Build history of the part. All positions in model axes, mm. Face numbers are marked on the shaded views. A direction names the side the tool comes from. Give positions to 0.01 mm unless a question says otherwise; leave off trailing zeros. Use a Markdown table: item, result. Add a question column.
(1) Flat gauge pins, fed straight in: pin 1 (2 mm diameter, centred on x = 70.5, y = -4.5, fed in from -Z) (3 decimals); pin 2 (1 mm diameter, centred on x = 233.5, z = -1, fed in from +Y). Where does each tip first touch, or does it go through?
(2) Which spindle directions (+Z, -Z, +X, -X, +Y, -Y) get a long thin tool onto all of the face, cutting with end or side? Do the marked faces 1 and 2. Say none if no direction does.
(3) Wall check: line 1 (Y direction, x = 650, z = -1.55); line 2 (Y direction, x = 520, z = -0.65); line 3 (Z direction, x = 351, y = 52.5) (3 decimals). Give the ranges that are in metal, low to high.
from build123d import *

# Parameters (mm, degrees)
SKETCH1_R                    = 11.9875
SKETCH1_R_2                  = 11.1125
SKETCH1_W                    = 75
SKETCH1_H                    = 10.02
BASE_FLANGE1_DEPTH           = 3.175
EDGE_FLANGE1_STRIP_W         = 14.1732
EDGE_FLANGE1_STRIP_H         = 3.175
EDGE_FLANGE1_STRIP_CUT_DEPTH = 910
EDGE_FLANGE1_DEPTH           = 910
M5_CLEARANCE_HOLE1_D         = 5.3
CUT_EXTRUDE2_REACH           = 784.448
FILLET1_R                    = 2
FILLET2_R                    = 5


# Sheet-metal steps are written as plain solids
with BuildPart() as part:
    # Sketch1 → Base-Flange1 (new body)
    with BuildSketch(Plane.XY):
        Polygon((-130, 60), (780, 60), (780, -20), (700, -55), (0, -55), (-130, -20), align=None)
        Circle(SKETCH1_R, mode=Mode.SUBTRACT)
        with Locations((183.333333333, 0)):
            Circle(SKETCH1_R, mode=Mode.SUBTRACT)
        with Locations((366.666666667, 0)):
            Circle(SKETCH1_R, mode=Mode.SUBTRACT)
        with Locations((550, 0)):
            Circle(SKETCH1_R, mode=Mode.SUBTRACT)
        with Locations((-110, 0)):
            Circle(SKETCH1_R_2, mode=Mode.SUBTRACT)
        with Locations((727.5, 0)):
            Rectangle(SKETCH1_W, SKETCH1_H, mode=Mode.SUBTRACT)
    extrude(amount=-BASE_FLANGE1_DEPTH)

    # Edge-Flange1 strip (across the edge) → Edge-Flange1 strip cut (cut)
    with BuildSketch(Plane(origin=(-130, 60, -3.175), x_dir=(0, -1, 0), z_dir=(1, 0, 0))):
        with Locations((-3.175, -1.5875)):
            Rectangle(EDGE_FLANGE1_STRIP_W, EDGE_FLANGE1_STRIP_H)
    extrude(amount=EDGE_FLANGE1_STRIP_CUT_DEPTH, mode=Mode.SUBTRACT)

    # Edge-Flange1 section (across the edge) → Edge-Flange1 (add)
    with BuildSketch(Plane(origin=(-130, 60, -3.175), x_dir=(0, -1, 0), z_dir=(1, 0, 0))):
        with BuildLine():
            Line((0, 0.7366), (0, 11.825))
            Line((0, 11.825), (3.175, 11.825))
            Line((3.175, 11.825), (3.175, 0.7366))
            ThreePointArc((3.175, 0.7366), (3.390745145, 0.215745145), (3.9116, 0))
            Line((3.9116, 0), (3.9116, -3.175))
            ThreePointArc((3.9116, -3.175), (1.145681115, -2.029318885), (0, 0.7366))
        make_face()
    extrude(amount=EDGE_FLANGE1_DEPTH)

    # M5 Clearance Hole1 (through all)
    with Locations(Plane(origin=(-50, 10, 0), x_dir=(1, 0, 0), z_dir=(0, 0, 1))):
        with Locations((0, 0), (0, -20), (20, -35), (20, 15), (183.333333333, 0), (183.333333333, -20), (203.333333333, -35), (203.333333333, 15), (366.666666667, 0), (366.666666667, -20), (386.666666667, -35), (386.666666667, 15), (550, 0), (550, -20), (570, -35), (570, 15), (700, 0), (700, -20), (720, 15), (720, -35)):
            Hole(M5_CLEARANCE_HOLE1_D / 2)

    # Sketch8 → Cut-Extrude2 (cut, up to next)
    with BuildSketch(Plane.XY, mode=Mode.PRIVATE) as cut_extrude2_sk1:
        Polygon((55.816057945, 40), (25, 40), (25, -22.943437506), align=None)
    cut_extrude2_tool1 = extrude(cut_extrude2_sk1.sketch, amount=-CUT_EXTRUDE2_REACH, mode=Mode.PRIVATE) & part.part
    # Sketch8 → Cut-Extrude2 (cut, up to next)
    with BuildSketch(Plane.XY, mode=Mode.PRIVATE) as cut_extrude2_sk2:
        Polygon((64.166666667, -40), (33.350608721, -40), (64.166666667, 22.943437506), align=None)
    cut_extrude2_tool2 = extrude(cut_extrude2_sk2.sketch, amount=-CUT_EXTRUDE2_REACH, mode=Mode.PRIVATE) & part.part
    # Sketch8 → Cut-Extrude2 (cut, up to next)
    with BuildSketch(Plane.XY, mode=Mode.PRIVATE) as cut_extrude2_sk3:
        Polygon((79.166666667, -40), (79.166666667, 22.943437506), (109.982724612, -40), align=None)
    cut_extrude2_tool3 = extrude(cut_extrude2_sk3.sketch, amount=-CUT_EXTRUDE2_REACH, mode=Mode.PRIVATE) & part.part
    # Sketch8 → Cut-Extrude2 (cut, up to next)
    with BuildSketch(Plane.XY, mode=Mode.PRIVATE) as cut_extrude2_sk4:
        Polygon((118.333333333, 40), (118.333333333, -22.943437506), (87.517275388, 40), align=None)
    cut_extrude2_tool4 = extrude(cut_extrude2_sk4.sketch, amount=-CUT_EXTRUDE2_REACH, mode=Mode.PRIVATE) & part.part
    # Sketch8 → Cut-Extrude2 (cut, up to next)
    with BuildSketch(Plane.XY, mode=Mode.PRIVATE) as cut_extrude2_sk5:
        Polygon((239.149391279, 40), (208.333333333, -22.943437506), (208.333333333, 40), align=None)
    cut_extrude2_tool5 = extrude(cut_extrude2_sk5.sketch, amount=-CUT_EXTRUDE2_REACH, mode=Mode.PRIVATE) & part.part
    # Sketch8 → Cut-Extrude2 (cut, up to next)
    with BuildSketch(Plane.XY, mode=Mode.PRIVATE) as cut_extrude2_sk6:
        Polygon((247.5, 22.943437506), (247.5, -40), (216.683942055, -40), align=None)
    cut_extrude2_tool6 = extrude(cut_extrude2_sk6.sketch, amount=-CUT_EXTRUDE2_REACH, mode=Mode.PRIVATE) & part.part
    # Sketch8 → Cut-Extrude2 (cut, up to next)
    with BuildSketch(Plane.XY, mode=Mode.PRIVATE) as cut_extrude2_sk7:
        Polygon((293.316057945, -40), (262.5, -40), (262.5, 22.943437506), align=None)
    cut_extrude2_tool7 = extrude(cut_extrude2_sk7.sketch, amount=-CUT_EXTRUDE2_REACH, mode=Mode.PRIVATE) & part.part
    # Sketch8 → Cut-Extrude2 (cut, up to next)
    with BuildSketch(Plane.XY, mode=Mode.PRIVATE) as cut_extrude2_sk8:
        Polygon((270.850608721, 40), (301.666666667, 40), (301.666666667, -22.943437506), align=None)
    cut_extrude2_tool8 = extrude(cut_extrude2_sk8.sketch, amount=-CUT_EXTRUDE2_REACH, mode=Mode.PRIVATE) & part.part
    # Sketch8 → Cut-Extrude2 (cut, up to next)
    with BuildSketch(Plane.XY, mode=Mode.PRIVATE) as cut_extrude2_sk9:
        Polygon((422.482724612, 40), (391.666666667, -22.943437506), (391.666666667, 40), align=None)
    cut_extrude2_tool9 = extrude(cut_extrude2_sk9.sketch, amount=-CUT_EXTRUDE2_REACH, mode=Mode.PRIVATE) & part.part
    # Sketch8 → Cut-Extrude2 (cut, up to next)
    with BuildSketch(Plane.XY, mode=Mode.PRIVATE) as cut_extrude2_sk10:
        Polygon((430.833333333, 22.943437506), (430.833333333, -40), (400.017275388, -40), align=None)
    cut_extrude2_tool10 = extrude(cut_extrude2_sk10.sketch, amount=-CUT_EXTRUDE2_REACH, mode=Mode.PRIVATE) & part.part
    # Sketch8 → Cut-Extrude2 (cut, up to next)
    with BuildSketch(Plane.XY, mode=Mode.PRIVATE) as cut_extrude2_sk11:
        Polygon((476.649391279, -40), (445.833333333, -40), (445.833333333, 22.943437506), align=None)
    cut_extrude2_tool11 = extrude(cut_extrude2_sk11.sketch, amount=-CUT_EXTRUDE2_REACH, mode=Mode.PRIVATE) & part.part
    # Sketch8 → Cut-Extrude2 (cut, up to next)
    with BuildSketch(Plane.XY, mode=Mode.PRIVATE) as cut_extrude2_sk12:
        Polygon((454.183942055, 40), (485, 40), (485, -22.943437506), align=None)
    cut_extrude2_tool12 = extrude(cut_extrude2_sk12.sketch, amount=-CUT_EXTRUDE2_REACH, mode=Mode.PRIVATE) & part.part
    # Sketch8 → Cut-Extrude2 (cut, up to next)
    with BuildSketch(Plane.XY, mode=Mode.PRIVATE) as cut_extrude2_sk13:
        Polygon((605.816057945, 40), (575, -22.943437506), (575, 40), align=None)
    cut_extrude2_tool13 = extrude(cut_extrude2_sk13.sketch, amount=-CUT_EXTRUDE2_REACH, mode=Mode.PRIVATE) & part.part
    # Sketch8 → Cut-Extrude2 (cut, up to next)
    with BuildSketch(Plane.XY, mode=Mode.PRIVATE) as cut_extrude2_sk14:
        Polygon((614.166666667, 22.943437506), (614.166666667, -40), (583.350608721, -40), align=None)
    cut_extrude2_tool14 = extrude(cut_extrude2_sk14.sketch, amount=-CUT_EXTRUDE2_REACH, mode=Mode.PRIVATE) & part.part
    # Sketch8 → Cut-Extrude2 (cut, up to next)
    with BuildSketch(Plane.XY, mode=Mode.PRIVATE) as cut_extrude2_sk15:
        Polygon((633.350608721, 40), (622.517275388, 40), (614.166666667, 22.943437506), (614.166666667, -40), (633.350608721, -40), align=None)
    cut_extrude2_tool15 = extrude(cut_extrude2_sk15.sketch, amount=-CUT_EXTRUDE2_REACH, mode=Mode.PRIVATE) & part.part
    add(cut_extrude2_tool1.solids().sort_by_distance((35.272019, 19.018854, 0))[0], mode=Mode.SUBTRACT)
    add(cut_extrude2_tool2.solids().sort_by_distance((53.894647, -19.018854, 0))[0], mode=Mode.SUBTRACT)
    add(cut_extrude2_tool3.solids().sort_by_distance((89.438686, -19.018854, 0))[0], mode=Mode.SUBTRACT)
    add(cut_extrude2_tool4.solids().sort_by_distance((108.061314, 19.018854, 0))[0], mode=Mode.SUBTRACT)
    add(cut_extrude2_tool5.solids().sort_by_distance((218.605353, 19.018854, 0))[0], mode=Mode.SUBTRACT)
    add(cut_extrude2_tool6.solids().sort_by_distance((237.227981, -19.018854, 0))[0], mode=Mode.SUBTRACT)
    add(cut_extrude2_tool7.solids().sort_by_distance((272.772019, -19.018854, 0))[0], mode=Mode.SUBTRACT)
    add(cut_extrude2_tool8.solids().sort_by_distance((291.394647, 19.018854, 0))[0], mode=Mode.SUBTRACT)
    add(cut_extrude2_tool9.solids().sort_by_distance((401.938686, 19.018854, 0))[0], mode=Mode.SUBTRACT)
    add(cut_extrude2_tool10.solids().sort_by_distance((420.561314, -19.018854, 0))[0], mode=Mode.SUBTRACT)
    add(cut_extrude2_tool11.solids().sort_by_distance((456.105353, -19.018854, 0))[0], mode=Mode.SUBTRACT)
    add(cut_extrude2_tool12.solids().sort_by_distance((474.727981, 19.018854, 0))[0], mode=Mode.SUBTRACT)
    add(cut_extrude2_tool13.solids().sort_by_distance((585.272019, 19.018854, 0))[0], mode=Mode.SUBTRACT)
    add(cut_extrude2_tool14.solids().sort_by_distance((603.894647, -19.018854, 0))[0], mode=Mode.SUBTRACT)
    add(cut_extrude2_tool15.solids().sort_by_distance((624.089948, -1.669801, 0))[0], mode=Mode.SUBTRACT)

    # Fillet1
    fillet1_edges = [part.edges().sort_by_distance(p)[0] for p in [
        (247.5, 22.943437506, -1.5875),
        (247.5, -40, -1.5875),
        (216.683942055, -40, -1.5875),
        (293.316057945, -40, -1.5875),
        (262.5, -40, -1.5875),
        (262.5, 22.943437506, -1.5875),
        (270.850608721, 40, -1.5875),
        (301.666666667, 40, -1.5875),
        (301.666666667, -22.943437506, -1.5875),
        (422.482724612, 40, -1.5875),
        (391.666666667, -22.943437506, -1.5875),
        (391.666666667, 40, -1.5875),
        (64.166666667, -40, -1.5875),
        (33.350608721, -40, -1.5875),
        (690, -5.01, -1.5875),
        (64.166666667, 22.943437506, -1.5875),
        (690, 5.01, -1.5875),
        (79.166666667, -40, -1.5875),
        (79.166666667, 22.943437506, -1.5875),
        (109.982724612, -40, -1.5875),
        (765, 5.01, -1.5875),
        (118.333333333, 40, -1.5875),
        (118.333333333, -22.943437506, -1.5875),
        (87.517275388, 40, -1.5875),
        (765, -5.01, -1.5875),
        (239.149391279, 40, -1.5875),
        (208.333333333, -22.943437506, -1.5875),
        (208.333333333, 40, -1.5875),
        (633.350608721, -40, -1.5875),
        (583.350608721, -40, -1.5875),
        (622.517275388, 40, -1.5875),
        (633.350608721, 40, -1.5875),
        (430.833333333, 22.943437506, -1.5875),
        (430.833333333, -40, -1.5875),
        (400.017275388, -40, -1.5875),
        (476.649391279, -40, -1.5875),
        (445.833333333, -40, -1.5875),
        (445.833333333, 22.943437506, -1.5875),
        (454.183942055, 40, -1.5875),
        (485, 40, -1.5875),
        (485, -22.943437506, -1.5875),
        (605.816057945, 40, -1.5875),
        (575, -22.943437506, -1.5875),
        (575, 40, -1.5875),
        (25, 40, -1.5875),
        (55.816057945, 40, -1.5875),
        (25, -22.943437506, -1.5875),
    ]]
    fillet(fillet1_edges, radius=FILLET1_R)

    # Fillet2
    fillet2_edges = [part.edges().sort_by_distance(p)[0] for p in [
        (780, -20, -1.5875),
        (700, -55, -1.5875),
        (0, -55, -1.5875),
        (-130, -20, -1.5875),
        (-130, 58.4125, -15),
        (780, 58.4125, -15),
    ]]
    fillet(fillet2_edges, radius=FILLET2_R)


solid = part.part
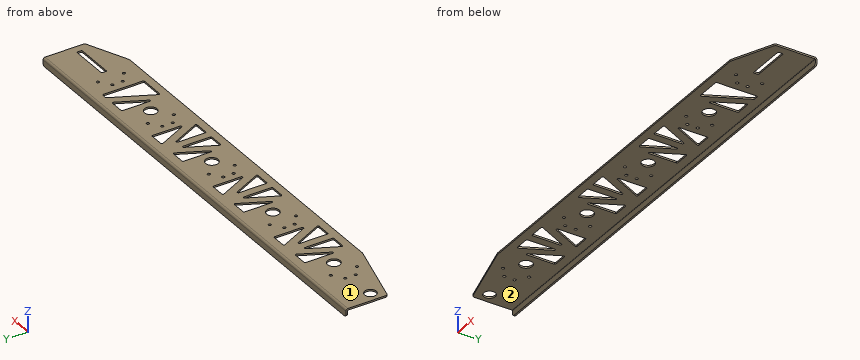
Solution:
| question | item | result |
|---|---|---|
| 1 | pin 1 | z = -3.175 |
| 1 | pin 2 | y = 59.17 |
| 2 | face 1 | +Z, +X, -X, +Y, -Y |
| 2 | face 2 | -Z, +X, -X, -Y |
| 3 | line 1 | -55 to -12.65, -7.35 to 7.35, 12.65 to 59.21 |
| 3 | line 2 | -55 to -27.65, -22.35 to 22.35, 27.65 to 58.25 |
| 3 | line 3 | -3.175 to 0 |
